Autodesk Inventor part; units mm, degrees
ref_plane "YZ Plane" through (0, 0, 0) normal (1, 0, 0) x (0, 1, 0)
ref_plane "XZ Plane" through (0, 0, 0) normal (0, 1, 0) x (-1, 0, 0)
ref_plane "XY Plane" through (0, 0, 0) normal (0, 0, 1) x (1, 0, 0)
ref_plane "Work Plane2" through (4.5, -13.125, 5) normal (0, 0, 1) x (1, 0, 0)
sketch "Sketch5" plane through (4.5, -13.125, 5) normal (0, 0, 1) x (1, 0, 0)
  circle A0 centre (-5.3843, -10.9183) radius 3.5
  line L0 (40.5, 19.8795) -> (20.6391, 19.8795)
  line L1 (20.6391, 19.8795) -> (-0.5, 15.425)
  line L2 (-0.5, 15.425) -> (-8.5, 15.425)
  line L3 (-8.5, 15.425) -> (-8.5, 12.625)
  line L4 (-8.5, 12.625) -> (-22.6946, 12.625)
  line L5 (-22.6946, 12.625) -> (-28.1392, 19.0495)
  arc A1 (-28.1392, 19.0495) -> (-34.556, 17.8156) centre (-31, 16.625) ccw
  spline S0 degree 3 poles (-34.556, 17.8156) (-34.7591, 16.8991) (-35.0888, 16.002) (-36.0242, 14.6392) (-36.5194, 14.1543) (-37.6005, 13.4479) (-38.1283, 13.21) (-39.2688, 12.8371) (-39.8866, 12.7101) (-40.5, 12.625) knots 0 0 0 0 0.281642 0.281642 0.494296 0.494296 0.667567 0.667567 0.853113 0.853113 0.853113 0.853113
  line L6 (-40.5, 12.625) -> (-40.5, 2.625)
  line L7 (-40.5, 2.625) -> (-0.5, 2.625)
  line L8 (-0.5, 2.625) -> (20.6391, 7.0795)
  line L9 (20.6391, 7.0795) -> (20.6391, -0.375)
  line L10 (20.6391, -0.375) -> (-19.5, -0.375)
  line L11 (-19.5, -0.375) -> (-19.5, -6.375)
  line L12 (-19.5, -6.375) -> (-16.1781, -6.375)
  line L13 (-16.1781, -6.375) -> (-16.1781, -20.375)
  line L14 (-16.1781, -20.375) -> (5.3645, -20.375)
  line L15 (5.3645, -20.375) -> (5.3645, -6.375)
  line L16 (5.3645, -6.375) -> (40.5, -6.375)
  line L17 (40.5, -6.375) -> (40.5, 19.8795)
  line L18 (20.6391, 19.3686) -> (20.6391, 7.5905)
  line L19 (20.6391, 7.5905) -> (17.9999, 7.0344)
  line L20 (17.9999, 7.0344) -> (17.2782, 10.4592)
  line L21 (17.2782, 10.4592) -> (2.6006, 7.3662)
  line L22 (2.6006, 7.3662) -> (3.3222, 3.9414)
  line L23 (3.3222, 3.9414) -> (-0.5, 3.136)
  line L24 (-0.5, 3.136) -> (-0.5, 14.914)
  line L25 (-0.5, 14.914) -> (2.9614, 15.6434)
  line L26 (2.9614, 15.6434) -> (3.6831, 12.2186)
  line L27 (3.6831, 12.2186) -> (18.3608, 15.3116)
  line L28 (18.3608, 15.3116) -> (17.6391, 18.7364)
  line L29 (17.6391, 18.7364) -> (20.6391, 19.3686)
  circle A2 centre (-4.5, 7.625) radius 1.4
  circle A3 centre (-4.5, 12.625) radius 1.4
  circle A4 centre (-19.5, 7.625) radius 1.4
  circle A5 centre (-34.5, 7.625) radius 1.4
  circle A6 centre (-31, 16.625) radius 1.5
  line L30 (-0.5, 2.625) -> (-0.5, 15.425)
  line L31 (-22.6946, 12.625) -> (-40.5, 12.625)
  arc A7 (-22.5, 30.625) -> (-8.5, 15.425) centre (-8.0073, 29.9262) ccw
  line L32 (-22.5, 30.625) -> (-40.5, 30.625)
  line L33 (-40.5, 30.625) -> (-40.5, 2.625)
  circle A8 centre (-31, 27.1712) radius 1.4
  point P0 (-4.5, 13.125)
extrude "Extrusion3" add sketch "Sketch5" along normal blind 10 contours L30 L24 L7 L6 L31 L4 L3 L2 | L3 L4 L5 A1 S0 L33 L32 A7 | L31 S0 A1 L5
sketch "Sketch6" plane through (4.5, -13.125, 15) normal (0, 0, 1) x (1, 0, 0)
  circle A0 centre (-34.5, 7.625) radius 1.4
  circle A1 centre (-19.5, 7.625) radius 1.4
  circle A2 centre (-4.5, 12.625) radius 1.4
  circle A3 centre (-4.5, 7.625) radius 1.4
  line L0 (-0.5, 15.425) -> (-8.5, 15.425)
  line L1 (-40.5, 30.625) -> (-40.5, 2.625)
  line L2 (-40.5, 2.625) -> (-0.5, 2.625)
  line L3 (-0.5, 2.625) -> (-0.5, 15.425)
  circle A4 centre (4.9975, 34.5751) radius 13.9 construction
  line L4 (-0.5, 2.625) -> (-0.5, 15.425)
  arc A5 (-0.5, 15.425) -> (13.6114, 16.6099) centre (4.9975, 34.5751) ccw
  line L5 (-8.5, 12.625) -> (-40.5, 12.625)
  line L6 (-40.5, 12.625) -> (-40.5, 34.5751)
  line L7 (-40.5, 34.5751) -> (-14.9261, 34.5751)
  line L8 (13.6114, 16.6099) -> (13.6114, -54.1295)
  line L9 (13.6114, 16.6099) -> (84.3508, 16.6099) construction
  line L10 (13.6114, -54.1295) -> (-40.5, -54.1295)
  line L11 (-40.5, -54.1295) -> (-40.5, 2.625)
  arc A6 (-22.5, 30.625) -> (-8.5, 15.425) centre (-8.0073, 29.9262) ccw
  line L12 (-22.5, 30.625) -> (-40.5, 30.625)
  circle A7 centre (-8.0073, 29.9262) radius 14.5095
  line L13 (-40.5, 30.625) -> (-40.5, 2.625)
  line L14 (-40.5, 30.625) -> (-40.5, 40.6638)
  line L15 (-8.0073, 44.4357) -> (-8.0073, 46.4357)
  line L16 (-8.0073, 46.4357) -> (-40.5, 46.4357)
  line L17 (-40.5, 46.4357) -> (-40.5, 30.625)
  line L18 (-22.5, 30.625) -> (-40.5, 30.625)
  line L19 (-22.5, 30.625) -> (-40.5, 30.625)
  point P0 (-4.5, 13.125)
  dimension "d15" = 90
  dimension "d25" = 2
  dimension "d26" = 90
extrude "Extrusion4" add sketch "Sketch6" along normal blind 7 contours L3 L2 L1 L12 A6 A7 L0 | A5 L8 L10 L11 L2 L3 | A7 L0
sketch "Sketch7" plane through (4.5, -13.125, 22) normal (0, 0, 1) x (1, 0, 0)
  circle A0 centre (-19.5, 7.625) radius 1.4
  circle A1 centre (-34.5, 7.625) radius 1.4
  circle A2 centre (-4.5, 7.625) radius 1.4
  circle A3 centre (-4.5, 12.625) radius 1.4
  circle A4 centre (-31, 16.625) radius 1.5
  circle A5 centre (-4.5, 7.625) radius 1.4
  circle A6 centre (-4.5, 12.625) radius 1.4
  circle A7 centre (-19.5, 7.625) radius 1.4
  circle A8 centre (-34.5, 7.625) radius 1.4
  line L0 (-0.5, 15.425) -> (-8.5, 15.425)
  arc A9 (-22.5, 30.625) -> (-8.5, 15.425) centre (-8.0073, 29.9262) ccw
  line L1 (-22.5, 30.625) -> (-40.5, 30.625)
  line L2 (-40.5, 30.625) -> (-40.5, -54.1295)
  line L3 (-40.5, -54.1295) -> (13.6114, -54.1295)
  line L4 (13.6114, -54.1295) -> (13.6114, 16.6099)
  arc A10 (-0.5, 15.425) -> (13.6114, 16.6099) centre (4.9975, 34.5751) ccw
  circle A11 centre (-31, 27.1712) radius 1.4
  circle A12 centre (-7, -33.875) radius 1.95
  point P0 (-4.5, 13.125)
hole "Hole2" at (-30, -5.5, 22) at (-15, -5.5, 22) at (0, -5.5, 22) at (0, -0.5, 22) at (-26.5, 3.5, 22) at (-2.5, -47, 22) at (-26.5, 14.0462, 22) direction (0, 0, -1) diameter 2.9 end through all counterbore diameter 7 counterbore depth 4
properties part number "cellSTORM_cellphone_plate"
Input: part model. Units: mm. Frame: model coordinates. A direction names the side the tool comes from. Round coordinates to 2 decimals unless told otherwise and drop trailing zeros. Loops run counter-clockwise (first coordinate to the right, second up) from the corner with the lowest first, then second, coordinate; pieces in that order, holes last. Notation, with made-up numbers: (30, 47.5) -> (40, 47.5) arc R24 ccw to (40, 59.5) -> close; hole circle Ø6 at (44.5, 88.25). An arc over 180 degrees is marked (long way). Answer as a JSON object with one key per item and string values. Group by question number.
1) Pin query (flat end, axial travel): pin 1 (7.5 mm diameter, centred on x = -25, y = 14, fed in from +Z); pin 2 (4.5 mm diameter, centred on x = -15, y = -5.5, fed in from +Z); pin 3 (3 mm diameter, centred on x = -25.5, z = 11, fed in from -Y); pin 4 (8 mm diameter, centred on x = -10.5, y = -48, fed in from -Z). Return the tip coordinate at first contact, or that it passes through.
2) Section query B-B on z = 10. Output: boundary loops of the cut face in (x, y).
3) Section query A-A on y = -47. Output: boundary loops of the cut face in (x, z), plus the area to 3 significant figures.
4) Ray query, L1, parallel to X at y = -5.5, z = 14.75; L2, parallel to Y at x = -26.5, z = 16.9; L3, parallel to X at y = -5.5, z = 21.05. Return the intervals inside material, ascending.
5) Reachability of faces 1 (the cylindrical face through (-11.895, -7.115, 19.972)), 2 (the cylindrical face through (-2.56, -45.55, 16.48)) from +Z, -Z, +X, -X, +Y, -Y: full face, straight path, thin tool, end or side. Return the list, or none.
6) Section query D-D on x = 0. Output: boundary loops of the cut face in (y, z).
7) Section query C-C on y = -5.5. State how many separate pieces and enclosed holes the cut face has, plus the area to 3 significant figures.
8) Draft query along X for faces 3 (the flat face through (18.111, -31, 18)), 4 (the flat face through (-27, 17.5, 13)), 5 (the flat face through (-28, -5, 18)). Return one class per face: +X half, -X half, draft (parallel to the pull), parting line (faces both ways), or undercut.
Reply:
{
 "1": {"pin 1": "stops at z = 22", "pin 2": "stops at z = 18", "pin 3": "stops at y = -10.5", "pin 4": "stops at z = 15"},
 "2": {"outline": "(-36, -10.5) -> (4, -10.5) -> (4, 2.3) -> (-4, 2.3) arc R14.51 cw to (-18, 17.5) -> (-36, 17.5) -> close; hole circle Ø2.9 at (-30, -5.5); hole circle Ø3 at (-26.5, 3.5); hole circle Ø2.9 at (-26.5, 14.05); hole circle Ø2.9 at (-15, -5.5); hole circle Ø2.9 at (0, -5.5); hole circle Ø2.9 at (0, -0.5)"},
 "3": {"outline": "(-36, 15) -> (-3.95, 15) -> (-3.95, 18) -> (-6, 18) -> (-6, 22) -> (-36, 22) -> close; (-1.05, 15) -> (18.11, 15) -> (18.11, 22) -> (1, 22) -> (1, 18) -> (-1.05, 18) -> close", "area": "342 mm2"},
 "4": {"L1": "x = -36 to -31.45, -28.55 to -16.45, -13.55 to -1.45, 1.45 to 4", "L2": "y = -67.25 to 2.05, 4.95 to 12.6, 15.5 to 17.5", "L3": "x = -36 to -33.5, -26.5 to -18.5, -11.5 to -3.5, 3.5 to 18.11"},
 "5": {"face 1": "+Z", "face 2": "+Z, -Z"},
 "6": {"outline": "(-67.25, 15) -> (-10.5, 15) -> (-10.5, 5) -> (-6.95, 5) -> (-6.95, 18) -> (-9, 18) -> (-9, 22) -> (-44.55, 22) -> (-44.55, 18) -> (-49.45, 18) -> (-49.45, 22) -> (-67.25, 22) -> close; (-4.05, 5) -> (-1.95, 5) -> (-1.95, 18) -> (-4.05, 18) -> close; (0.95, 5) -> (2.3, 5) -> (2.3, 18) -> (0.95, 18) -> close"},
 "7": {"separate pieces": "4", "enclosed holes": "0", "area": "582 mm2"},
 "8": {"face 3": "+X half", "face 4": "draft", "face 5": "undercut"}
}
